Here's the drawing with two shaded views (mm, measured from the low corner). I have some questions. A direction names the side the tool comes from. Give positions to 0.01 mm unless a question says otherwise; leave off trailing zeros. Write each loop counter-clockwise with the first axis right and the second up, starting at its lowest first coordinate (ties: lowest second). Pieces come first, ordered by that corner, then holes. Notation, with made-up numbers: (-11.75, 3.25) -> (43.25, 3.25) arc R35 cw to (43.25, 36.25) -> close; hole circle Ø2 at (15, 46.25). An arc over 180 degrees is marked (long way). One line per item, written item: value.
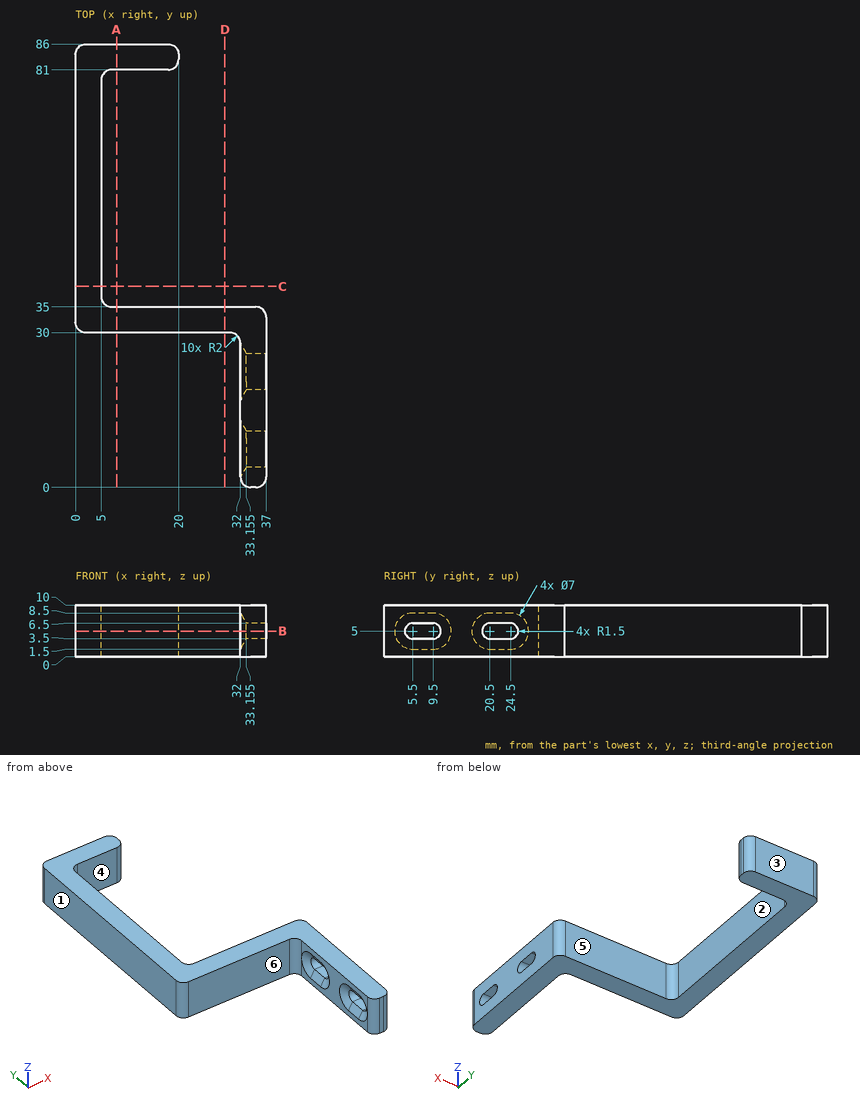
1) If we section it at A-A (x = 8): Write out the boundary of the cut face in (y, z).
Answer list:
outline: (30, 0) -> (35, 0) -> (35, 10) -> (30, 10) -> close; (81, 0) -> (86, 0) -> (86, 10) -> (81, 10) -> close
2) If we section it at D-D (x = 29): Write out the boundary of the cut face in (y, z).
Answer list:
outline: (30, 0) -> (35, 0) -> (35, 10) -> (30, 10) -> close
3) I need wall thicknesses on L1, parallel to Y at x = 13.5, z = 7; L2, parallel to Y at x = 35, z = 2; L3, parallel to Y at x = 23, z = 4.75. Which ranges of each line are inside material? Lowest first, please.
Answer list:
L1: y = 30 to 35, 81 to 86
L2: y = 0 to 35
L3: y = 30 to 35
4) For the marked faces 1 and 2, which set-ups out of +Z, -Z, +X, -X, +Y, -Y let a thin tool reach every point of the face, with its end or its side?
Answer list:
face 1: +Z, -Z, -X, +Y, -Y
face 2: +Z, -Z, +X
5) If we section it at B-B (z = 5): State how many separate pieces and enclosed holes the cut face has, and give its area (3 significant figures).
Answer list:
separate pieces: 3
enclosed holes: 0
area: 587 mm^2
6) If we section it at C-C (y = 39): Write out the boundary of the cut face in (x, z), and give its area (3 significant figures).
Answer list:
outline: (0, 0) -> (5, 0) -> (5, 10) -> (0, 10) -> close
area: 50.0 mm^2
7) We'd pull the mould along Y, two halves only. Please class the marked faces 3, 4, 5 and 6: released by +Y, released by -Y, zero draft, split by the parting line, or undercut.
Answer list:
face 3: released by +Y
face 4: undercut
face 5: undercut
face 6: released by -Y
8) Will these pins go through, and if not, where does the flat tip stop? pin 1 (1 mm diameter, centred on x = 7.5, z = 8.5, fed in from -Y); pin 2 (1 mm diameter, centred on x = 32, z = 6.5, fed in from -Y); pin 3 (3 mm diameter, centred on x = 22, z = 7, fed in from +Y).
Answer list:
pin 1: stops at y = 30
pin 2: stops at y = 0.68
pin 3: stops at y = 35
